Autodesk Inventor part; units mm, degrees
ref_plane "YZ Plane" through (0, 0, 0) normal (1, 0, 0) x (0, 1, 0)
ref_plane "XZ Plane" through (0, 0, 0) normal (0, 1, 0) x (-1, 0, 0)
ref_plane "XY Plane" through (0, 0, 0) normal (0, 0, 1) x (1, 0, 0)
sketch "Skizze1" plane through (0, 0, 0) normal (0, 1, 0) x (-1, 0, 0)
  line L0 (-20, 20) -> (20, 20)
  line L1 (20, 20) -> (20, -20)
  line L2 (20, -20) -> (-20, -20)
  line L3 (-20, -20) -> (-20, 20)
  circle A0 centre (0, 0) radius 13.5
  dimension "d0" = 40
  dimension "d1" = 40
  dimension "d2" = 27
  dimension "d16" = 20
extrude "Extrusion1" add sketch "Skizze1" against normal blind 0.2
sketch "Skizze2" plane through (0, -0.2, 0) normal (0, -1, 0) x (1, 0, 0)
  point P0 (0, 0)
  point P1 (-16, -16)
  point P2 (-16, 16)
  point P3 (16, -16)
  point P4 (16, 16)
  dimension "d12" = 32
  dimension "d13" = 16
  dimension "d14" = 32
  dimension "d15" = 16
hole "Bohrung1" at (-16, -0.2, -16) at (-16, -0.2, 16) at (16, -0.2, -16) at (16, -0.2, 16) direction (0, 1, 0) diameter 2.459 depth 0.2
properties part number "zylinderfussdichtung"
Could you check a few things on this model? Use its own coordinates, in mm. Round coordinates to 2 decimals unless told otherwise and drop trailing zeros. Loops run counter-clockwise (first coordinate to the right, second up) from the corner with the lowest first, then second, coordinate; pieces in that order, holes last. Notation, with made-up numbers: (84.5, -9.5) - (138.5, -9.5) arc R21 cw to (138.5, 27.5) - close; hole circle Ø9 at (1.25, 83). An arc over 180 degrees is marked (long way). Answer in a Markdown table with one row per item. Add a question column.
(1) If we section it at A-A (x = 16): Please give me the cut outline in (y, z).
(2) If we section it at C-C (x = 0): Please give me the cut outline in (y, z), plus the area to 3 significant figures.
(3) If we section it at D-D (y = -0.05): Please give me the cut outline in (x, z).
(4) If we section it at B-B (z = -16): Please give me the cut outline in (x, y), plus the area to 3 significant figures.
(5) I need wall thicknesses on line 1 along X through (y, z) = (-0.1, -16); line 2 along Z through (x, y) = (0, -0.1); line 3 along Z through (x, y) = (-7, -0.1). Which ranges of each line are inside material? Lowest first, please.
Model answer:
| question | item | result |
|---|---|---|
| 1 | outline | (-0.2, -20) - (0, -20) - (0, -17.23) - (-0.2, -17.23) - close; (-0.2, -14.77) - (0, -14.77) - (0, 14.77) - (-0.2, 14.77) - close; (-0.2, 17.23) - (0, 17.23) - (0, 20) - (-0.2, 20) - close |
| 2 | outline | (-0.2, -20) - (0, -20) - (0, -13.5) - (-0.2, -13.5) - close; (-0.2, 13.5) - (0, 13.5) - (0, 20) - (-0.2, 20) - close |
| 2 | area | 2.60 mm² |
| 3 | outline | (-20, -20) - (20, -20) - (20, 20) - (-20, 20) - close; hole circle Ø2.46 at (-16, -16); hole circle Ø2.46 at (-16, 16); hole circle Ø27 at (0, 0); hole circle Ø2.46 at (16, -16); hole circle Ø2.46 at (16, 16) |
| 4 | outline | (-20, -0.2) - (-17.23, -0.2) - (-17.23, 0) - (-20, 0) - close; (-14.77, -0.2) - (14.77, -0.2) - (14.77, 0) - (-14.77, 0) - close; (17.23, -0.2) - (20, -0.2) - (20, 0) - (17.23, 0) - close |
| 4 | area | 7.02 mm² |
| 5 | line 1 | x = -20 to -17.23, -14.77 to 14.77, 17.23 to 20 |
| 5 | line 2 | z = -20 to -13.5, 13.5 to 20 |
| 5 | line 3 | z = -20 to -11.54, 11.54 to 20 |
